For this review, take the finished solid that the model builds, in its own axes (mm). Face numbers are marked on the shaded views. A direction names the side the tool comes from. Give positions to 0.01 mm unless a question says otherwise; leave off trailing zeros. Order: outer loops, then holes, each group sorted by start corner. A loop starts at its lowest first (then second) coordinate and runs counter-clockwise, first axis right, second up. Notation, with made-up numbers: (39, -18) - (72, -18) arc R16 ccw to (72, 3) - close; hole circle Ø3 at (-17.75, 2.5). An arc over 180 degrees is marked (long way). Answer as a JSON object with one key per item and string values. Group by question number.
from build123d import *

# Parameters (mm, degrees)
SKETCH4_R           = 3.96875
SKETCH4_R_2         = 3.175
BOSS_EXTRUDE2_DEPTH = 10.16
FILLET1_R           = 3.81


with BuildPart() as part:
    # Sketch4 → Boss-Extrude2 (new body)
    with BuildSketch(Plane(origin=(0, 0, 0), x_dir=(1, 0, 0), z_dir=(0, 1, 0))):
        with BuildLine():
            Line((54.2925, 31.75), (-12.3825, 31.75))
            Line((-12.3825, 31.75), (-7.863361559, -1.082336008))
            ThreePointArc((-7.863361559, -1.082336008), (-3.056289676, -7.325503373), (4.7625, -6.35))
            Line((4.7625, -6.35), (41.91, -6.35))
            ThreePointArc((41.91, -6.35), (45.967580476, -4.884520517), (48.152310263, -1.164501002))
            Line((48.152310263, -1.164501002), (54.2925, 31.75))
        make_face()
        with Locations(Location((0, 0, 0), (0, 0, 270))):
            Circle(SKETCH4_R, mode=Mode.SUBTRACT)
        with Locations(Location((46.355, 22.86, 0), (0, 0, 270))):
            Circle(SKETCH4_R, mode=Mode.SUBTRACT)
        with Locations(Location((-4.445, 22.86, 0), (0, 0, 270))):
            Circle(SKETCH4_R, mode=Mode.SUBTRACT)
        with Locations(Location((41.91, 0, 0), (0, 0, 270))):
            Circle(SKETCH4_R_2, mode=Mode.SUBTRACT)
        with BuildLine():
            Line((36.730478204, 29.21), (6.985, 29.21))
            ThreePointArc((6.985, 29.21), (5.188948776, 28.466051224), (4.445, 26.67))
            Line((4.445, 26.67), (4.445, 8.043333333))
            ThreePointArc((4.445, 8.043333333), (5.188948776, 6.247282109), (6.985, 5.503333333))
            Line((6.985, 5.503333333), (33.255679437, 5.503333333))
            ThreePointArc((33.255679437, 5.503333333), (34.878711627, 6.089525126), (35.752603542, 7.577532932))
            Line((35.752603542, 7.577532932), (39.227402309, 26.204199599))
            ThreePointArc((39.227402309, 26.204199599), (38.684286411, 28.29303219), (36.730478204, 29.21))
        make_face(mode=Mode.SUBTRACT)
        with BuildLine():
            Line((46.58698696, 4.295147609), (48.631735848, 15.256028661))
            ThreePointArc((48.631735848, 15.256028661), (44.519378774, 15.137668683), (40.900146495, 17.093850549))
            Line((40.900146495, 17.093850549), (38.737442476, 5.500670755))
            ThreePointArc((38.737442476, 5.500670755), (42.873923491, 6.276412312), (46.58698696, 4.295147609))
        make_face(mode=Mode.SUBTRACT)
        with BuildLine():
            Line((36.83, -3.81), (6.963318623, -3.81))
            ThreePointArc((6.963318623, -3.81), (7.800370345, -1.469057088), (7.872207457, 1.016))
            Line((7.872207457, 1.016), (35.641806959, 1.016))
            ThreePointArc((35.641806959, 1.016), (35.744131016, -1.518077625), (36.83, -3.81))
        make_face(mode=Mode.SUBTRACT)
        with BuildLine():
            Line((-6.14066773, 5.029523445), (-7.591897143, 15.572960504))
            ThreePointArc((-7.591897143, 15.572960504), (-3.525796009, 14.975903966), (0.293891225, 16.492361803))
            Line((0.293891225, 16.492361803), (1.490851578, 7.796234208))
            ThreePointArc((1.490851578, 7.796234208), (-2.705340953, 7.462240721), (-6.14066773, 5.029523445))
        make_face(mode=Mode.SUBTRACT)
    extrude(amount=BOSS_EXTRUDE2_DEPTH)

    # Fillet1
    fillet1_edges = [part.edges().sort_by_distance(p)[0] for p in [
        (-12.3825, 5.08, -31.75),
        (54.2925, 5.08, -31.75),
    ]]
    fillet(fillet1_edges, radius=FILLET1_R)


solid = part.part
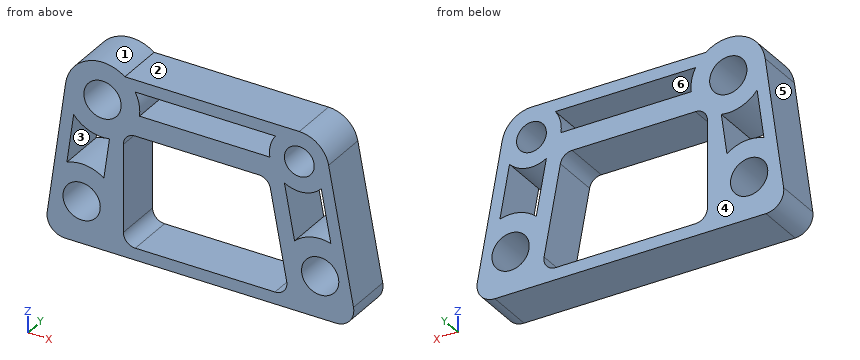
1) Consider section C-C (y = 6.25). Give the number of separate pieces and of enclosed holes in the cut face, plus the area to 3 significant figures.
2) Consider section D-D (x = 5.5). Give the boundary of the cut face in (y, z).
3) Consider section A-A (x = 13). Give the boundary of the cut face in (y, z).
4) For the marked faces 1, 2 and 3, list the 3-axis set-ups (+Z, -Z, +X, -X, +Y, -Y) from which the entire face can be reached by the end or side of a thin tool; tool diameter is ignored.
5) Mouldability with a two-part tool opening along Z and no side actions: class the marked faces 4, 5 and 6 as released by +Z, released by -Z, zero draft, split by the parting line, or undercut.
6) For line 1 (Z direction, x = 9, y = 8); line 2 (X direction, y = 8, z = -10.5) (1 decimal); line 3 (X direction, y = 9, z = -22) (3 decimals), list the stretches that pass through material, from the lowest coordinate up.
7) For pin 1 (7 mm diameter, centred on x = 46.355, z = -22.86, fed in from +Y); pin 2 (6 mm diameter, centred on y = 1, z = -11.5, fed in from +X); pin 3 (5 mm diameter, centred on x = 21, y = 7.5, fed in from +Z); pin 4 (4 mm diameter, centred on y = 3.5, z = -14.5, fed in from -X), all flat-tipped, find the tip position at first contact; note any pin that passes through.
8) Consider section B-B (z = -13). Give the boundary of the cut face in (x, y) (3 decimals).
Result set:
{
 "1": {"separate pieces": "1", "enclosed holes": "8", "area": "1,060 mm2"},
 "2": {"outline": "(0, -31.75) - (10.16, -31.75) - (10.16, -28.73) - (0, -28.73) - close; (0, -5.98) - (10.16, -5.98) - (10.16, 6.35) - (0, 6.35) - close"},
 "3": {"outline": "(0, -31.75) - (10.16, -31.75) - (10.16, -29.21) - (0, -29.21) - close; (0, -5.5) - (10.16, -5.5) - (10.16, -1.02) - (0, -1.02) - close; (0, 3.81) - (10.16, 3.81) - (10.16, 6.35) - (0, 6.35) - close"},
 "4": {"face 1": "+Z, +Y, -Y", "face 2": "+Z, +X, +Y, -Y", "face 3": "+Y, -Y"},
 "5": {"face 4": "zero draft", "face 5": "released by +Z", "face 6": "undercut"},
 "6": {"line 1": "z = -31.75 to -29.21, -5.5 to -1.02, 3.81 to 6.35", "line 2": "x = -9.5 to -6.9, 1.1 to 4.4, 36.3 to 39.7, 47.7 to 50.3", "line 3": "x = -11.04 to -8.319, -0.571 to 4.445, 38.443 to 42.481, 50.229 to 52.474"},
 "7": {"pin 1": "passes through", "pin 2": "stops at x = 51.07", "pin 3": "stops at z = 6.35", "pin 4": "stops at x = -10.28"},
 "8": {"outline": "(-9.802, 0) - (-7.238, 0) - (-7.238, 10.16) - (-9.802, 10.16) - close; (0.775, 0) - (4.445, 0) - (4.445, 10.16) - (0.775, 10.16) - close; (36.764, 0) - (40.136, 0) - (40.136, 10.16) - (36.764, 10.16) - close; (48.211, 0) - (50.795, 0) - (50.795, 10.16) - (48.211, 10.16) - close"}
}
